Could you check a few things on this model? Use its own coordinates, in mm. A direction names the side the tool comes from. Give positions to 0.01 mm unless a question says otherwise; leave off trailing zeros. Order: outer loops, then holes, each group sorted by start corner. A loop starts at its lowest first (then second) coordinate and runs counter-clockwise, first axis right, second up.
from build123d import *

# Parameters (mm, degrees)
BOSS_EXTRUDE1_DEPTH            = 12
SKETCH41_R                     = 1.7
CUT_EXTRUDE7_DEPTH             = 18
CBORE_FOR_M3_SHCS1_D           = 3.4
CBORE_FOR_M3_SHCS1_CBORE_D     = 6.5
CBORE_FOR_M3_SHCS1_CBORE_DEPTH = 3
F_3DSKETCH3_START              = 9
F_3DSKETCH3_OUTLINE_R          = 3.25
F_3DSKETCH3_OUTLINE_R_2        = 1.7
F_3DSKETCH3_DEPTH              = 3
CUT_EXTRUDE10_DEPTH            = 15
CUT_EXTRUDE10_DEPTH_BACK       = 15
SKETCH52_R                     = 1.7
SKETCH58_R                     = 3.25
CUT_EXTRUDE11_DEPTH            = 8
CUT_EXTRUDE12_DEPTH            = 4
CUT_EXTRUDE12_DEPTH_BACK       = 6
FILLET1_R                      = 2
SKETCH61_R                     = 3.25
CUT_EXTRUDE13_DEPTH            = 6
CUT_EXTRUDE14_DEPTH            = 1


# Read off the part's stored shape, not the designer's step: 3DSketch3
with BuildPart() as part:
    # Sketch1 → Boss-Extrude1 (new body)
    with BuildSketch(Plane(origin=(0, 0, 0), x_dir=(0, 1, 0), z_dir=(0, 0, 1))):
        with BuildLine():
            Line((-6.350852961, -13), (13.279056191, -13))
            Line((13.279056191, -13), (13.279056191, -1))
            Line((13.279056191, -1), (3.97617907, -1))
            ThreePointArc((3.97617907, -1), (3.650947901, -1.865631106), (3.14, -2.636361129))
            Line((3.14, -2.636361129), (-3.14, -2.636361129))
            ThreePointArc((-3.14, -2.636361129), (-3.852531635, -1.402854233), (-4.1, 0))
            ThreePointArc((-4.1, 0), (-0.503818326, 4.06892702), (3.97617907, 1))
            Line((3.97617907, 1), (13.279056191, 1))
            Line((13.279056191, 1), (13.279056191, 13))
            Line((13.279056191, 13), (-6.350852961, 13))
            Line((-6.350852961, 13), (-13.856406461, 0))
            Line((-13.856406461, 0), (-6.350852961, -13))
        make_face()
    extrude(amount=BOSS_EXTRUDE1_DEPTH)

    # Sketch41 → Cut-Extrude7 (cut)
    with BuildSketch(Plane(origin=(0, 0, 0), x_dir=(0, 1, 0), z_dir=(0, 0, 1))):
        with Locations(Location((0, 8.6, 0), (0, 0, 270))):
            Circle(SKETCH41_R)
        with Locations(Location((0, -8.6, 0), (0, 0, 270))):
            Circle(SKETCH41_R)
    extrude(amount=CUT_EXTRUDE7_DEPTH, mode=Mode.SUBTRACT)

    # CBORE for M3 SHCS1 (through all)
    with Locations(Plane(origin=(-8.6, 0, 12), x_dir=(1, 0, 0), z_dir=(0, 0, 1))):
        with Locations((0, 0)):
            CounterBoreHole(CBORE_FOR_M3_SHCS1_D / 2, CBORE_FOR_M3_SHCS1_CBORE_D / 2, CBORE_FOR_M3_SHCS1_CBORE_DEPTH)

    # 3DSketch3 outline → 3DSketch3 (cut)
    with BuildSketch(Plane.XY.offset(F_3DSKETCH3_START)):
        with Locations((8.6, 0)):
            Circle(F_3DSKETCH3_OUTLINE_R)
        with Locations((8.6, 0)):
            Circle(F_3DSKETCH3_OUTLINE_R_2, mode=Mode.SUBTRACT)
    extrude(amount=F_3DSKETCH3_DEPTH, mode=Mode.SUBTRACT)

    # Sketch52 → Cut-Extrude10 (cut, two sides: drawn at the far end of the back side and taken through both)
    with BuildSketch(Plane.YZ.offset(-1).offset(-CUT_EXTRUDE10_DEPTH_BACK)):
        with Locations((8.106406461, 6)):
            Circle(SKETCH52_R)
    extrude(amount=CUT_EXTRUDE10_DEPTH + CUT_EXTRUDE10_DEPTH_BACK, mode=Mode.SUBTRACT)

    # Sketch58 → Cut-Extrude11 (cut)
    with BuildSketch(Plane.YZ.offset(13)):
        with Locations(Location((8.106406461, 6, 0), (0, 0, 270))):
            Circle(SKETCH58_R)
    extrude(amount=-CUT_EXTRUDE11_DEPTH, mode=Mode.SUBTRACT)

    # Sketch60 → Cut-Extrude12 (cut, two sides: drawn at the far end of the back side and taken through both)
    with BuildSketch(Plane.YZ.offset(-8).offset(-CUT_EXTRUDE12_DEPTH_BACK)):
        Polygon((8.106406461, 2.709103466), (10.956406461, 4.354551733), (10.956406461, 7.645448267), (8.106406461, 9.290896534), (5.256406461, 7.645448267), (5.256406461, 4.354551733), align=None)
    extrude(amount=CUT_EXTRUDE12_DEPTH + CUT_EXTRUDE12_DEPTH_BACK, mode=Mode.SUBTRACT)

    # Fillet1
    # the kernel refuses this fillet: 2 mm, written as the material it takes off along each edge
    with BuildSketch(Plane(origin=(13, 13.279056191, -5), x_dir=(0, -1, 0), z_dir=(0, 0, 1)), Plane(origin=(-13, 13.279056191, -5), x_dir=(1, 0, 0), z_dir=(0, 0, 1))) as fillet1_piece_1:
        with BuildLine():
            CenterArc((FILLET1_R, -FILLET1_R), FILLET1_R, 90, 90)
            Line((0, -FILLET1_R), (0, 0))
            Line((0, 0), (FILLET1_R, 0))
        make_face()
    extrude(amount=22, mode=Mode.SUBTRACT)

    # Sketch61 → Cut-Extrude13 (cut)
    with BuildSketch(Plane(origin=(0, 0, 12), x_dir=(0, 1, 0), z_dir=(0, 0, 1))):
        with Locations(Location((0, 8.6, 0), (0, 0, 270))):
            Circle(SKETCH61_R)
        with Locations(Location((0, -8.6, 0), (0, 0, 270))):
            Circle(SKETCH61_R)
    extrude(amount=-CUT_EXTRUDE13_DEPTH, mode=Mode.SUBTRACT)

    # Sketch62 → Cut-Extrude14 (cut)
    with BuildSketch(Plane(origin=(-6, -10.392304845, 0), x_dir=(-0.8660254037844386, 0.5000000000000001, 0), z_dir=(-0.5000000000000001, -0.8660254037844386, 0))):
        with BuildLine():
            Line((1.32365953, -3.245174166), (1.009556966, -3.245174166))
            add(Edge.make_bspline(
                [(1.009556966, -3.245174166), (1.011604119, -3.203503278), (1.015624673, -3.121662763), (1.034452962, -3.002338857), (1.061393839, -2.888284058), (1.099485293, -2.780414144), (1.146791571, -2.677775337), (1.203521598, -2.580775321), (1.270715449, -2.489784132), (1.346922183, -2.405645289), (1.429690822, -2.328457718), (1.518996761, -2.261802476), (1.612841789, -2.205484804), (1.710941188, -2.158403562), (1.814401751, -2.123063716), (1.922284609, -2.096842077), (2.035063745, -2.081065731), (2.111903767, -2.079369946), (2.150983248, -2.078507499)],
                knots=[0, 0, 0, 0, 1.10065271, 2.161652631, 3.183658789, 4.190468796, 5.17591951, 6.163126047, 7.15150782, 8.156236427, 9.156009102, 10.134482811, 11.092018607, 12.041330605, 13.001268258, 13.972401359, 14.968799086, 16, 16, 16, 16], degree=3))
            add(Edge.make_bspline(
                [(2.150983248, -2.078507499), (2.189361322, -2.079405955), (2.264772866, -2.08117139), (2.374834881, -2.096332419), (2.479612175, -2.120078011), (2.578899942, -2.153393427), (2.671906006, -2.198177855), (2.759329051, -2.251975393), (2.842209862, -2.314195225), (2.916816645, -2.387449038), (2.985324725, -2.465651423), (3.04442698, -2.549139326), (3.095040143, -2.635368612), (3.137227823, -2.724996814), (3.168283962, -2.818867842), (3.19186217, -2.915615045), (3.205189584, -3.016239856), (3.207235007, -3.084346411), (3.208274914, -3.118972242)],
                knots=[0, 0, 0, 0, 1.111607364, 2.184268762, 3.212621178, 4.221274766, 5.211760367, 6.196651075, 7.1921475, 8.207485113, 9.220403448, 10.201281604, 11.166441695, 12.114753415, 13.065576456, 14.026450734, 14.996634279, 16, 16, 16, 16], degree=3))
            add(Edge.make_bspline(
                [(3.208274914, -3.118972242), (3.206588269, -3.167722052), (3.203244578, -3.26436618), (3.174388875, -3.406570537), (3.129806778, -3.544475597), (3.075733749, -3.655454649), (3.021113181, -3.744431542), (2.972933386, -3.818347183), (2.915281033, -3.8971736), (2.84868362, -3.981704709), (2.774145813, -4.072199079), (2.691131146, -4.168693845), (2.599005455, -4.27016415), (2.534347273, -4.339469963), (2.500843023, -4.375382499)],
                knots=[0, 0, 0, 0, 1.184203166, 2.347625244, 3.513805382, 4.700623107, 5.337941753, 6.051866363, 6.845199593, 7.711357327, 8.668078039, 9.695487809, 10.805859518, 12, 12, 12, 12], degree=3))
            Line((2.500843023, -4.375382499), (1.625141902, -5.30927673))
            Line((1.625141902, -5.30927673), (3.253146709, -5.30927673))
            Line((3.253146709, -5.30927673), (3.253146709, -5.668251089))
            Line((3.253146709, -5.668251089), (0.874941581, -5.668251089))
            Line((0.874941581, -5.668251089), (2.232313376, -4.21973346))
            add(Edge.make_bspline(
                [(2.232313376, -4.21973346), (2.265361263, -4.185235154), (2.32883949, -4.118970967), (2.418622067, -4.022228007), (2.499261055, -3.932478466), (2.571278448, -3.849891918), (2.633111953, -3.77326035), (2.687984185, -3.705065647), (2.731949776, -3.642311196), (2.779665172, -3.569570582), (2.825879153, -3.480758265), (2.865591509, -3.372224576), (2.889806358, -3.260497323), (2.892711193, -3.184995286), (2.89417235, -3.147017114)],
                knots=[0, 0, 0, 0, 1.329631726, 2.553950428, 3.673215718, 4.687767853, 5.603093632, 6.413772471, 7.123043292, 7.734684054, 8.834405432, 9.900288307, 10.943827018, 12, 12, 12, 12], degree=3))
            add(Edge.make_bspline(
                [(2.89417235, -3.147017114), (2.893536608, -3.123135716), (2.892283682, -3.076070065), (2.881225984, -3.007064306), (2.864515478, -2.940499493), (2.84057022, -2.876170874), (2.80896348, -2.814725221), (2.7704901, -2.756087741), (2.726100037, -2.699398776), (2.674748768, -2.646245478), (2.618337248, -2.597564273), (2.558742998, -2.554440187), (2.495692894, -2.518401076), (2.429452772, -2.488857579), (2.360207302, -2.465682198), (2.287822557, -2.449623619), (2.212498541, -2.439541135), (2.161065045, -2.438176963), (2.134857446, -2.437481858)],
                knots=[0, 0, 0, 0, 0.991446411, 1.95395049, 2.89581595, 3.838931463, 4.798493298, 5.75982156, 6.748411868, 7.785213223, 8.824556874, 9.840280684, 10.836137867, 11.835679398, 12.848801643, 13.863922112, 14.911575587, 16, 16, 16, 16], degree=3))
            add(Edge.make_bspline(
                [(2.134857446, -2.437481858), (2.107486614, -2.43819689), (2.053734817, -2.439601095), (1.974815784, -2.449423759), (1.899530007, -2.4663696), (1.827688104, -2.489546274), (1.759168518, -2.519004823), (1.694304474, -2.555696568), (1.633241585, -2.599480061), (1.575865062, -2.649120617), (1.523001082, -2.704388218), (1.476554207, -2.765998181), (1.435970192, -2.832825597), (1.400560959, -2.904690147), (1.371805269, -2.982243927), (1.349832118, -3.065211632), (1.332445272, -3.153233014), (1.326636751, -3.214018099), (1.32365953, -3.245174166)],
                knots=[0, 0, 0, 0, 1.031018746, 2.02475058, 2.990194455, 3.934040569, 4.864654155, 5.795059489, 6.735614925, 7.690564532, 8.649604399, 9.611025574, 10.590972636, 11.591080095, 12.624614302, 13.701020113, 14.821632451, 16, 16, 16, 16], degree=3))
        make_face()
    extrude(amount=-CUT_EXTRUDE14_DEPTH, mode=Mode.SUBTRACT)


solid = part.part
Item 1: We'd pull the mould along Z, two halves only. Please class faces 6 (the flat face through (-13, 3, 6)), 7 (the cylindrical face through (9.056, 5.223, 4.5)), 8 (the flat face through (3, 3, 12)): +Z half, -Z half, draft (parallel to the pull), parting line (faces both ways), or undercut.
Findings:
face 6: draft
face 7: undercut
face 8: +Z half
Item 2: Imagine slicing it at C-C on x = 2.25. List the corners of the cut face in (y, z) for me, then the cut area to 3 significant figures.
Findings:
outline: (-12.56, 0) - (-3.43, 0) - (-3.43, 12) - (-12.56, 12) - close; (3.43, 0) - (13.28, 0) - (13.28, 12) - (3.43, 12) - close; hole circle Ø3.4 at (8.11, 6)
area: 219 mm2
Item 3: For faces 1 (the flat face through (-7.545, -8.931, 4.836)), 2 (the cylindrical face through (1.85, 3.66, 5.92)), 3 (the cylindrical face through (12.43, 12.68, 5.92)), 4 (the flat face through (-8.563, 9.551, 8.457)), 5 (the flat face through (5, 6.7, 4.6)), which set-ups out of +Z, -Z, +X, -X, +Y, -Y let a thin tool reach every point of the face, with its end or its side?
Findings:
face 1: none
face 2: +Z, -Z
face 3: +Z, -Z, +X, +Y
face 4: -X
face 5: +X
Item 4: Imagine slicing it at D-D on y = -10.75. List the corners of the cut face in (x, z) for me, then the cut area to 3 significant figures.
Findings:
outline: (-5.38, 0) - (5.38, 0) - (5.38, 12) - (-5.38, 12) - close
area: 129 mm2
Item 5: For pin 1 (1.6 mm diameter, centred on x = -6.5, z = 6.5, fed in from -Y); pin 2 (1.5 mm diameter, centred on y = -7.5, z = 8, fed in from +X); pin 3 (6 mm diameter, centred on x = 8.6, y = 0, fed in from +Z), each with a flat end and sliding along its axis, tell me the tip position at first contact or that it passes through.
Findings:
pin 1: stops at y = -10.57
pin 2: stops at x = 12.31
pin 3: stops at z = 6
Item 6: Please list where these lines run through material, in increasing order: line 1 along X through (y, z) = (9.5, 1.75); line 2 along Z through (x, y) = (4.25, 8.25); line 3 along Y through (x, z) = (-1.85, 6).
Findings:
line 1: x = -13 to -1, 1 to 13
line 2: z = 0 to 4.31, 7.69 to 12
line 3: y = -12.79 to -3.66, 3.66 to 6.41, 9.81 to 13.28
Item 7: Imagine slicing it at B-B on y = 0. List the corners of the cut face in (x, z) for me, then the cut area to 3 significant figures.
Findings:
outline: (-13, 0) - (-10.3, 0) - (-10.3, 6) - (-11.85, 6) - (-11.85, 12) - (-13, 12) - close; (-6.9, 0) - (-4.1, 0) - (-4.1, 12) - (-5.35, 12) - (-5.35, 6) - (-6.9, 6) - close; (2.64, 0) - (6.9, 0) - (6.9, 6) - (5.35, 6) - (5.35, 12) - (2.64, 12) - close; (10.3, 0) - (13, 0) - (13, 12) - (11.85, 12) - (11.85, 6) - (10.3, 6) - close
area: 112 mm2
Item 8: Imagine slicing it at A-A on x = 8.6. List the corners of the cut face in (y, z) for me.
Findings:
outline: (-8.89, 0) - (-1.7, 0) - (-1.7, 6) - (-3.25, 6) - (-3.25, 12) - (-8.89, 12) - close; (1.7, 0) - (13.28, 0) - (13.28, 12) - (3.25, 12) - (3.25, 6) - (1.7, 6) - close; hole circle Ø6.5 at (8.11, 6)
